Check sheet for the modelled part. Datum: model origin and axes. Units: mm. A direction names the side the tool comes from. Round coordinates to 2 decimals unless told otherwise and drop trailing zeros. Write each loop counter-clockwise with the first axis right and the second up, starting at its lowest first coordinate (ties: lowest second). Pieces come first, ordered by that corner, then holes.
Autodesk Inventor part; units mm, degrees
ref_plane "YZ Plane" through (0, 0, 0) normal (1, 0, 0) x (0, 1, 0)
ref_plane "XZ Plane" through (0, 0, 0) normal (0, 1, 0) x (-1, 0, 0)
ref_plane "XY Plane" through (0, 0, 0) normal (0, 0, 1) x (1, 0, 0)
sketch "Sketch1" plane through (0, 0, 0) normal (0, 1, 0) x (-1, 0, 0)
  circle A0 centre (0, 0) radius 2.75
  dimension "d0" = 5.5
extrude "Extrusion1" add sketch "Sketch1" along normal blind 8.547
chamfer "Chamfer1" distance 0.4 angle 45 1 edges at (2.75, 8.547, 0)
sketch "Sketch2" plane through (0, 8.547, 0) normal (0, 1, 0) x (1, 0, 0)
  circle A0 centre (0, 0) radius 2.35
  circle A1 centre (0, 0) radius 0.75
  dimension "d6" = 1.5
extrude "Extrusion2" cut sketch "Sketch2" against normal blind 0.5 contours A1
properties part number "main_lcd_push_button" material "ABS Plastic"
1. Sectioned sample at B-B, the plane z = 0. Enter the section's corners in (x, y).
2. Set-up check for faces 1 (the flat face through (1, 8.547, 1)), 2 (the flat face through (0, 8.047, 0)): record each of +Z, -Z, +X, -X, +Y, -Y from which the full face is reachable in a straight line by a thin tool's end or side.
3. Release check for a two-part mould opening along X. For faces 3 (the cylindrical face through (-0.75, 8.3, -0.03)), 4 (the flat face through (0, 0, 0)), 5 (the cylindrical face through (0.596, 4.016, 2.685)) record: released by +X, released by -X, zero draft, split by the parting line, or undercut.
4. Go/stop test with flat-tipped pins: pin 1 (0.8 mm diameter, centred on x = 0, z = 0, fed in from +Y); pin 2 (1.5 mm diameter, centred on x = -1.5, y = 4, fed in from -Z). Record where each tip stops, or that it passes through.
5. Sectioned sample at C-C, the plane y = 3. Enter the section's corners in (x, z), plus the area to 3 significant figures.
6. Scan lines: line 1 along X through (y, z) = (8.2, 0); line 2 along Z through (x, y) = (0, 8.4); line 3 along Y through (x, z) = (-0.2, 0.25). Record each from-to range of solid material in increasing order.
7. Sectioned sample at A-A, the plane x = 0. Enter the section's corners in (y, z).
Computed values:
1. outline: (-2.75, 0) - (2.75, 0) - (2.75, 8.15) - (2.35, 8.55) - (0.75, 8.55) - (0.75, 8.05) - (-0.75, 8.05) - (-0.75, 8.55) - (-2.35, 8.55) - (-2.75, 8.15) - close
2. face 1: +Z, -Z, +X, -X, +Y
2. face 2: +Y
3. face 3: undercut
3. face 4: zero draft
3. face 5: split by the parting line
4. pin 1: stops at y = 8.05
4. pin 2: stops at z = -2.65
5. outline: circle Ø5.5 at (0, 0)
5. area: 23.8 mm2
6. line 1: x = -2.7 to -0.75, 0.75 to 2.7
6. line 2: z = -2.5 to -0.75, 0.75 to 2.5
6. line 3: y = 0 to 8.05
7. outline: (0, -2.75) - (8.15, -2.75) - (8.55, -2.35) - (8.55, -0.75) - (8.05, -0.75) - (8.05, 0.75) - (8.55, 0.75) - (8.55, 2.35) - (8.15, 2.75) - (0, 2.75) - close
